CAD build for the part. Positions are in the model's coordinates, mm. Face numbers are marked on the shaded views. Round coordinates to 2 decimals unless told otherwise and drop trailing zeros. Loops run counter-clockwise (first coordinate to the right, second up) from the corner with the lowest first, then second, coordinate; pieces in that order, holes last. Notation, with made-up numbers: (29.5, 86.5) - (44.5, 86.5) arc R27 cw to (44.5, 115.5) - close; hole circle Ø11 at (-30, 55). An arc over 180 degrees is marked (long way). One line per question, with ' | ' between items.
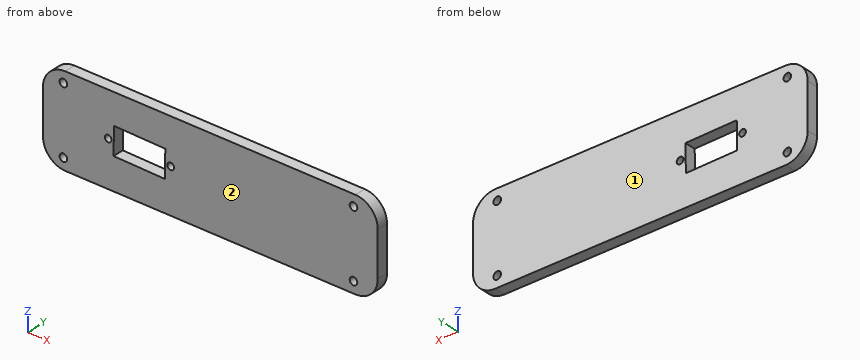
```python
from build123d import *

# Parameters (mm, degrees)
SKETCH9_W           = 150
SKETCH9_H           = 40
BOSS_EXTRUDE5_DEPTH = 5
SKETCH11_R          = 1.7
CUT_EXTRUDE6_DEPTH  = 103.952823134
FILLET1_R           = 10
SKETCH13_R          = 1.5
CUT_EXTRUDE7_DEPTH  = 103.952823134


with BuildPart() as part:
    # Sketch9 → Boss-Extrude5 (new body)
    with BuildSketch(Plane(origin=(0, 0, 0), x_dir=(1, 0, 0), z_dir=(0, 1, 0))):
        with Locations((25.867654831, 0)):
            Rectangle(SKETCH9_W, SKETCH9_H)
    extrude(amount=BOSS_EXTRUDE5_DEPTH)

    # Sketch11 → Cut-Extrude6 (cut, through all)
    with BuildSketch(Plane(origin=(0, 5, 0), x_dir=(1, 0, 0), z_dir=(0, 1, 0))):
        with Locations(Location((-40, 15, 0), (0, 0, 270))):
            Circle(SKETCH11_R)
        with Locations(Location((90, 15, 0), (0, 0, 270))):
            Circle(SKETCH11_R)
        with Locations(Location((90, -15, 0), (0, 0, 270))):
            Circle(SKETCH11_R)
        with Locations(Location((-40, -15, 0), (0, 0, 270))):
            Circle(SKETCH11_R)
    extrude(amount=-CUT_EXTRUDE6_DEPTH, mode=Mode.SUBTRACT)

    # Fillet1
    fillet1_edges = [part.edges().sort_by_distance(p)[0] for p in [
        (100.867654831, 2.5, 20),
        (-49.132345169, 2.5, 20),
        (-49.132345169, 2.5, -20),
        (100.867654831, 2.5, -20),
    ]]
    fillet(fillet1_edges, radius=FILLET1_R)

    # Sketch13 → Cut-Extrude7 (cut, through all)
    with BuildSketch(Plane.XZ):
        with Locations(Location((8.073804278, -0.138958576, 0), (0, 0, 270))):
            Circle(SKETCH13_R)
        with Locations(Location((-19.922049564, 0.342879212, 0), (0, 0, 270))):
            Circle(SKETCH13_R)
        Polygon((-17.527391561, -5.799238749), (-17.317447953, 6.398954711), (5.679146274, 6.003159385), (5.469202666, -6.195034075), align=None)
    extrude(amount=-CUT_EXTRUDE7_DEPTH, mode=Mode.SUBTRACT)


solid = part.part
```
(1) Drop a flat-ended pin along its axis: P1, Ø2, axis at y = 2, z = -14.5, coming from the +X side. Give the stop position or say it passes through.
Results found:
P1: stops at x = 100.24
(2) Probe L1, parallel to X at y = 4, z = -16.5; L2, parallel to X at y = 1.65, z = -15; L3, parallel to Z at x = 89.5, y = 4.15. List the from-to ranges inside material, lowest first.
Results found:
L1: x = -46.73 to -40.8, -39.2 to 89.2, 90.8 to 98.47 | L2: x = -47.79 to -41.7, -38.3 to 88.3, 91.7 to 99.53 | L3: z = -20 to -16.62, -13.38 to 13.38, 16.62 to 20
(3) Cut at B-B, the plane y = 1.55. Write the cut outline in (x, z).
Results found:
outline: (-49.13, -10) arc R10 ccw to (-39.13, -20) - (90.87, -20) arc R10 ccw to (100.87, -10) - (100.87, 10) arc R10 ccw to (90.87, 20) - (-39.13, 20) arc R10 ccw to (-49.13, 10) - close; hole circle Ø3.4 at (-40, -15); hole circle Ø3.4 at (-40, 15); hole circle Ø3 at (-19.92, 0.34); hole (-17.53, -5.8) - (5.47, -6.2) - (5.68, 6) - (-17.32, 6.4) - close; hole circle Ø3 at (8.07, -0.14); hole circle Ø3.4 at (90, -15); hole circle Ø3.4 at (90, 15)
(4) Cut at A-A, the plane z = -15. Write the cut outline in (x, y).
Results found:
outline: (-47.79, 0) - (-41.7, 0) - (-41.7, 5) - (-47.79, 5) - close; (-38.3, 0) - (88.3, 0) - (88.3, 5) - (-38.3, 5) - close; (91.7, 0) - (99.53, 0) - (99.53, 5) - (91.7, 5) - close
(5) Two-plate mould, pull along Y, no slides. Class the marked faces 1 and 2: released by +Y, released by -Y, zero draft, split by the parting line, or undercut.
Results found:
face 1: released by +Y | face 2: released by -Y
